from build123d import *

# Parameters (mm, degrees)
SKETCH_1_W                   = 100
SKETCH_1_H                   = 40
EXTRUDE_1_DEPTH              = 10
EXTRUDE_2_DEPTH              = 10
SKETCH_3_W                   = 40
SKETCH_3_H                   = 3
CUT_EXTRUDE_1_DEPTH          = 85.409715081
HOLE_WIZARD_M8_1_D           = 8.4
HOLE_WIZARD_M8_1_CBORE_D     = 18.01
HOLE_WIZARD_M8_1_CBORE_DEPTH = 5.68
FILLET_1_R                   = 8
FILLET_2_R                   = 3


with BuildPart() as part:
    # 스케치1 → 보스-돌출1 (new body)
    with BuildSketch(Plane(origin=(0, 0, 0), x_dir=(1, 0, 0), z_dir=(0, 1, 0))):
        with Locations((0, 20)):
            Rectangle(SKETCH_1_W, SKETCH_1_H)
    extrude(amount=EXTRUDE_1_DEPTH)

    # 스케치2 → 보스-돌출2 (add)
    with BuildSketch(Plane.XY):
        with BuildLine():
            Line((-20, 0), (-20, 35))
            ThreePointArc((-20, 35), (0, 55), (20, 35))
            Line((20, 35), (20, 0))
            Line((20, 0), (-20, 0))
        make_face()
    extrude(amount=-EXTRUDE_2_DEPTH)

    # 스케치3 → 컷-돌출1 (cut, through all)
    with BuildSketch(Plane.XY):
        with Locations((0, 1.5)):
            Rectangle(SKETCH_3_W, SKETCH_3_H)
    extrude(amount=-CUT_EXTRUDE_1_DEPTH, mode=Mode.SUBTRACT)

    # M8 육각 머리 볼트용 카운터보어1 (through all)
    with Locations(Plane(origin=(0, 35, 0), x_dir=(1, 0, 0), z_dir=(0, 0, 1))):
        with Locations((0, 0)):
            CounterBoreHole(HOLE_WIZARD_M8_1_D / 2, HOLE_WIZARD_M8_1_CBORE_D / 2, HOLE_WIZARD_M8_1_CBORE_DEPTH)

    # 필렛1
    fillet_1_edges = [part.edges().sort_by_distance(p)[0] for p in [
        (-50, 5, -40),
        (50, 5, -40),
        (50, 5, 0),
        (-50, 5, 0),
    ]]
    fillet(fillet_1_edges, radius=FILLET_1_R)

    # 필렛2
    fillet_2_edges = [part.edges().sort_by_distance(p)[0] for p in [
        (31, 10, 0),
        (-20, 22.5, -10),
        (20, 22.5, -10),
        (-20, 22.5, 0),
        (20, 22.5, 0),
        (0, 55, 0),
        (-20, 10, -5),
        (0, 55, -10),
        (20, 10, -5),
        (0, 10, -10),
        (-31, 10, 0),
        (-50, 10, -20),
        (50, 10, -20),
        (0, 10, -40),
        (47.656854249, 10, -37.656854249),
        (47.656854249, 10, -2.343145751),
        (-47.656854249, 10, -37.656854249),
        (-47.656854249, 10, -2.343145751),
    ]]
    fillet(fillet_2_edges, radius=FILLET_2_R)


solid = part.part
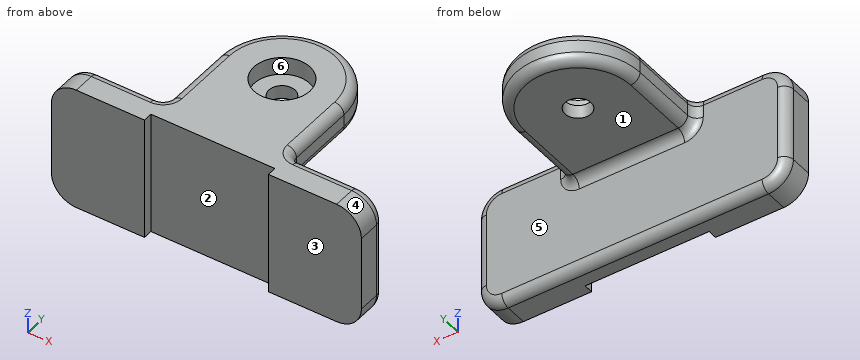
Verification items for the finished model (mm, model axes). Face numbers are marked on the shaded views. A direction names the side the tool comes from. Round coordinates to 2 decimals unless told otherwise and drop trailing zeros. Loops run counter-clockwise (first coordinate to the right, second up) from the corner with the lowest first, then second, coordinate; pieces in that order, holes last. Notation, with made-up numbers: (-2, 11.5) - (17, 11.5) arc R35 ccw to (17, 45.5) - close; hole circle Ø10 at (58.5, 21.5). An arc over 180 degrees is marked (long way). Answer in a Markdown table with one row per item. Add a question column.
Q1. Section check A-A on x = 0. Enter the section's corners in (y, z) (3 decimals).
Q2. Gauge pin test, flat ends, axial feed: pin 1 (1.5 mm diameter, centred on x = -37, z = -5.5, fed in from +Y); pin 2 (10 mm diameter, centred on y = 47, z = -5.5, fed in from +X) (3 decimals); pin 3 (6 mm diameter, centred on x = -17.5, y = 7.5, fed in from -Z); pin 4 (3 mm diameter, centred on y = 29.5, z = -4.5, fed in from +X). Record the tip position at first contact, or that the pin passes through.
Q3. Section check C-C on y = 18. Enter the section's corners in (x, z), plus the area to 3 significant figures.
Q4. Release check for a two-part mould opening along X. For the marked faces 4, 5 and 6 record: pulls with the +X half, pulls with the -X half, needs draft (parallel to the pull), parting line crosses it, or undercut.
Q5. Section check B-B on z = -19. Enter the section's corners in (x, y), plus the area to 3 significant figures.
Q6. Material ranges on line 1 (X direction, y = 2.5, z = -26); line 2 (Y direction, x = 20.5, z = -35); line 3 (Y direction, x = 0, z = -7.35), recorded low to high.
Q7. Section check D-D on x = -38. Enter the section's corners in (y, z), plus the area to 3 significant figures.
Q8. Tool access check on the marked faces 1, 2 and 3. Record the directions out of +Z, -Z, +X, -X, +Y, -Y that give a thin tool (end or side, any length) a straight path to the whole face; none if there is none.
Found:
| question | item | result |
|---|---|---|
| 1 | outline | (3, -40) - (7, -40) arc R3 ccw to (10, -37) - (10, -13) arc R3 cw to (13, -10) - (30.8, -10) - (30.8, -5.68) - (25.995, -5.68) - (25.995, 0) - (3, 0) - close; (39.2, -10) - (52, -10) arc R3 ccw to (55, -7) - (55, -3) arc R3 ccw to (52, 0) - (44.005, 0) - (44.005, -5.68) - (39.2, -5.68) - close |
| 2 | pin 1 | stops at y = 10 |
| 2 | pin 2 | stops at x = 18.735 |
| 2 | pin 3 | stops at z = -40 |
| 2 | pin 4 | stops at x = 20 |
| 3 | outline | (-20, -7) arc R3 ccw to (-17, -10) - (17, -10) arc R3 ccw to (20, -7) - (20, -3) arc R3 ccw to (17, 0) - (-17, 0) arc R3 ccw to (-20, -3) - close |
| 3 | area | 392 mm² |
| 4 | face 4 | pulls with the +X half |
| 4 | face 5 | needs draft |
| 4 | face 6 | undercut |
| 5 | outline | (-50, 0) - (-20, 0) - (-20, 3) - (20, 3) - (20, 0) - (50, 0) - (50, 7) arc R3 ccw to (47, 10) - (-47, 10) arc R3 ccw to (-50, 7) - close |
| 5 | area | 876 mm² |
| 6 | line 1 | x = -50 to -20, 20 to 50 |
| 6 | line 2 | y = 0 to 10 |
| 6 | line 3 | y = 3 to 30.8, 39.2 to 54.98 |
| 7 | outline | (0, -40) - (7, -40) arc R3 ccw to (10, -37) - (10, -3) arc R3 ccw to (7, 0) - (0, 0) - close |
| 7 | area | 396 mm² |
| 8 | face 1 | -Z, +X, -X, +Y |
| 8 | face 2 | +Z, -Z, -Y |
| 8 | face 3 | +Z, -Z, +X, -X, -Y |
